Source: CAD feature listing. Evaluate the final solid. Frame: model axes, mm. A direction names the side the tool comes from. Coordinates: 2 decimals unless noted, no trailing zeros. Order: outer loops, then holes, each group sorted by start corner. A loop starts at its lowest first (then second) coordinate and runs counter-clockwise, first axis right, second up. Notation, with made-up numbers: (-34, 25) - (-17, 25) arc R20 ccw to (-17, 38) - close; hole circle Ø10 at (56, -6.75). An arc over 180 degrees is marked (long way). One line per question, with ' | ' between items. Start each with the question number.
(1) Section D-D (z = -1.5). Return the cut outline in (x, y), then the cut area to 3 significant figures.
(2) Section B-B (z = -19). Return the cut outline in (x, y).
(3) Draft query along X for faces 1 (the flat face through (64.8, 5, -31.2)), 2 (the flat face through (69, 1.5, -15.3)), 3 (the flat face through (0, 3, -15)). Return one class per face: +X half, -X half, draft (parallel to the pull), parting line (faces both ways), or undercut.
(4) Line query: line 1 along X through (y, z) = (0.4, -29.5); line 2 along X through (y, z) = (3.05, -3); line 3 along Y through (x, z) = (49.5, -18.5). Output: solid intervals per line, ascending.
(5) Section A-A (y = 3). Return the cut outline in (x, z).
(6) Contact query for flat-ended pins moving along their axis: P1, Ø0.9, axis at x = 19.5, y = 3, coming from the -Z side; P2, Ø0.8, axis at y = 4.5, z = -23.5, coming from the -X side; P3, Ø0.8, axis at y = 4.5, z = -0.5, coming from the +X side. Output: stop coordinate, or through.
(7) Section C-C (x = 9.5). Return the cut outline in (y, z).
(8) Access query for faces 4 (the flat face through (67, 3, -2)), 5 (the flat face through (2, 2, -33)), 6 (the flat face through (68, 3, -5)), 7 (the flat face through (32, 1, -24.5)). Directions: +Z, -Z, +X, -X, +Y, -Y. A direction counts if a zero-diameter tool reaches every point of the face in a straight line with its end or side. Return the directions, or none.
from build123d import *

# Parameters (mm, degrees)
SKETCH1_W           = 71
SKETCH1_H           = 35
BOSS_EXTRUDE1_DEPTH = 2
SKETCH2_W           = 71
SKETCH2_H           = 35
SKETCH2_W_2         = 67
SKETCH2_H_2         = 31
BOSS_EXTRUDE2_DEPTH = 2
SKETCH3_W           = 69
SKETCH3_H           = 33
SKETCH3_W_2         = 67
SKETCH3_H_2         = 31
BOSS_EXTRUDE3_DEPTH = 1
SKETCH4_W           = 22
SKETCH4_H           = 3
CUT_EXTRUDE1_DEPTH  = 5
SKETCH5_W           = 53
SKETCH5_H           = 8.5
CUT_EXTRUDE2_DEPTH  = 5


with BuildPart() as part:
    # Sketch1 → Boss-Extrude1 (new body)
    with BuildSketch(Plane(origin=(0, 0, 0), x_dir=(1, 0, 0), z_dir=(0, 1, 0))):
        with Locations((33.5, 15.5)):
            Rectangle(SKETCH1_W, SKETCH1_H)
    extrude(amount=BOSS_EXTRUDE1_DEPTH)

    # Sketch2 → Boss-Extrude2 (add)
    with BuildSketch(Plane(origin=(0, 2, 0), x_dir=(1, 0, 0), z_dir=(0, 1, 0))):
        with Locations((33.5, 15.5)):
            Rectangle(SKETCH2_W, SKETCH2_H)
        with Locations((33.5, 15.5)):
            Rectangle(SKETCH2_W_2, SKETCH2_H_2, mode=Mode.SUBTRACT)
    extrude(amount=BOSS_EXTRUDE2_DEPTH)

    # Sketch3 → Boss-Extrude3 (add)
    with BuildSketch(Plane(origin=(0, 4, 0), x_dir=(1, 0, 0), z_dir=(0, 1, 0))):
        with Locations((33.5, 15.5)):
            Rectangle(SKETCH3_W, SKETCH3_H)
        with Locations((33.5, 15.5)):
            Rectangle(SKETCH3_W_2, SKETCH3_H_2, mode=Mode.SUBTRACT)
    extrude(amount=BOSS_EXTRUDE3_DEPTH)

    # Sketch4 → Cut-Extrude1 (cut)
    with BuildSketch(Plane.ZY.offset(-67)):
        with Locations((-16, 3.5)):
            Rectangle(SKETCH4_W, SKETCH4_H)
    extrude(amount=-CUT_EXTRUDE1_DEPTH, mode=Mode.SUBTRACT)

    # Sketch5 → Cut-Extrude2 (cut)
    with BuildSketch(Plane.XZ):
        with Locations((32.5, -28.75)):
            Rectangle(SKETCH5_W, SKETCH5_H)
    extrude(amount=-CUT_EXTRUDE2_DEPTH, mode=Mode.SUBTRACT)


solid = part.part
Response values:
1) outline: (-2, 0) - (69, 0) - (69, 4) - (68, 4) - (68, 5) - (67, 5) - (67, 2) - (0, 2) - (0, 5) - (-1, 5) - (-1, 4) - (-2, 4) - close | area: 152 mm²
2) outline: (-2, 0) - (69, 0) - (69, 2) - (0, 2) - (0, 5) - (-1, 5) - (-1, 4) - (-2, 4) - close
3) face 1: draft | face 2: +X half | face 3: undercut
4) line 1: x = -2 to 6, 59 to 69 | line 2: x = -2 to 0, 67 to 69 | line 3: y = 0 to 2
5) outline: (-2, -33) - (6, -33) - (6, -31) - (0, -31) - (0, 0) - (67, 0) - (67, -5) - (69, -5) - (69, 2) - (-2, 2) - close; (59, -33) - (69, -33) - (69, -27) - (67, -27) - (67, -31) - (59, -31) - close
6) P1: stops at z = 0 | P2: stops at x = -1 | P3: stops at x = 68
7) outline: (0, -24.5) - (2, -24.5) - (2, 0) - (5, 0) - (5, 1) - (4, 1) - (4, 2) - (0, 2) - close
8) face 4: +Y | face 5: -Z, +X, -X, +Y, -Y | face 6: +X, +Y | face 7: -Z, +Y, -Y
